```python
from build123d import *

# Parameters (mm, degrees)
SKETCH1_W           = 25.4
SKETCH1_H           = 25.4
SKETCH1_W_2         = 22.225
SKETCH1_H_2         = 22.225
BOSS_EXTRUDE1_DEPTH = 358.775
SKETCH4_R           = 2.54
CUT_EXTRUDE3_DEPTH  = 361.568746046


with BuildPart() as part:
    # Sketch1 → Boss-Extrude1 (new body)
    with BuildSketch(Plane.XY):
        with Locations((12.7, 12.7)):
            Rectangle(SKETCH1_W, SKETCH1_H)
        with Locations((12.7, 12.7)):
            Rectangle(SKETCH1_W_2, SKETCH1_H_2, mode=Mode.SUBTRACT)
    extrude(amount=BOSS_EXTRUDE1_DEPTH)

    # Sketch4 → Cut-Extrude3 (cut, through all)
    with BuildSketch(Plane(origin=(25.4, 0, 0), x_dir=(0, 0, -1), z_dir=(1, 0, 0))):
        with Locations((-350.8375, 12.7)):
            Circle(SKETCH4_R)
        with Locations((-325.4375, 12.7)):
            Circle(SKETCH4_R)
        with Locations((-300.0375, 12.7)):
            Circle(SKETCH4_R)
        with Locations(Location((-58.7375, 12.7, 0), (0, 0, 180))):
            Circle(SKETCH4_R)
        with Locations(Location((-33.3375, 12.7, 0), (0, 0, 180))):
            Circle(SKETCH4_R)
        with Locations(Location((-7.9375, 12.7, 0), (0, 0, 180))):
            Circle(SKETCH4_R)
        with Locations((-192.0875, 12.7)):
            Circle(SKETCH4_R)
        with Locations(Location((-166.6875, 12.7, 0), (0, 0, 180))):
            Circle(SKETCH4_R)
    extrude(amount=-CUT_EXTRUDE3_DEPTH, mode=Mode.SUBTRACT)


solid = part.part
```
Read the model definition and answer for the solid it produces. Units are mm, in the model's axes. A direction names the side the tool comes from. Give positions to 0.01 mm unless a question says otherwise; leave off trailing zeros. Order: outer loops, then holes, each group sorted by start corner. A loop starts at its lowest first (then second) coordinate and runs counter-clockwise, first axis right, second up. Notation, with made-up numbers: (-26.75, 20.5) -> (10.25, 20.5) arc R16 cw to (10.25, 30.5) -> close; hole circle Ø5 at (67.5, 64). An arc over 180 degrees is marked (long way). One line per item, written item: value. Start each with the question number.
(1) The part is cut by section A-A (x = 6). Determine the outline of the cut face in (y, z) (1 decimal), and give its area (3 significant figures).
(2) A straight line is drawn through the part: L1, parallel to Y at x = 10.75, z = 246. Find the intervals that lie inside material, in ascending order.
(3) A tool of negligible diameter and unlimited length cuts with its end or side. For faces 1 (the flat face through (13, 25.4, 177)), 2 (the flat face through (1.587, 13, 177)), from which of +Z, -Z, +X, -X, +Y, -Y can it reach the whole face along a straight path? Write none if from no direction.
(4) The part is cut by section B-B (z = 201). Determine the outline of the cut face in (x, y), and give its area (3 significant figures).
(5) For a pull along Y with two mould halves and no side action, classify faces 3 (the flat face through (13, 1.587, 177)), 4 (the flat face through (25.4, 13, 177)), 5 (the flat face through (13, 0, 177)), 6 (the flat face through (13, 23.812, 177)) as released by +Y, released by -Y, zero draft, split by the parting line, or undercut.
Taken from the geometry:
1. outline: (0, 0) -> (1.6, 0) -> (1.6, 358.8) -> (0, 358.8) -> close; (23.8, 0) -> (25.4, 0) -> (25.4, 358.8) -> (23.8, 358.8) -> close
1. area: 1,140 mm^2
2. L1: 0 to 1.59, 23.81 to 25.4
3. face 1: +Z, -Z, +X, -X, +Y
3. face 2: +Z, -Z
4. outline: (0, 0) -> (25.4, 0) -> (25.4, 25.4) -> (0, 25.4) -> close; hole (1.59, 1.59) -> (23.81, 1.59) -> (23.81, 23.81) -> (1.59, 23.81) -> close
4. area: 151 mm^2
5. face 3: undercut
5. face 4: zero draft
5. face 5: released by -Y
5. face 6: undercut
